from build123d import *

# Parameters (mm, degrees)
MODEL_R                 = 1.5
SALIENTE_EXTRUIR1_DEPTH = 3


with BuildPart() as part:
    # Model → Saliente-Extruir1 (new body)
    with BuildSketch(Plane.XY):
        with BuildLine():
            Line((256.429131311, 228.742243614), (355.429131311, 228.742243614))
            ThreePointArc((355.429131311, 228.742243614), (358.611111826, 227.424224129), (359.929131311, 224.242243614))
            Line((359.929131311, 224.242243614), (359.929131311, 215.242243614))
            ThreePointArc((359.929131311, 215.242243614), (358.611111826, 212.060263099), (355.429131311, 210.742243614))
            Line((355.429131311, 210.742243614), (256.429131311, 210.742243614))
            ThreePointArc((256.429131311, 210.742243614), (253.247150795, 212.060263099), (251.929131311, 215.242243614))
            Line((251.929131311, 215.242243614), (251.929131311, 224.242243614))
            ThreePointArc((251.929131311, 224.242243614), (253.247150795, 227.424224129), (256.429131311, 228.742243614))
        make_face()
        with Locations((337.429131311, 215.242243614)):
            Circle(MODEL_R, mode=Mode.SUBTRACT)
        with Locations((319.429131311, 215.242243614)):
            Circle(MODEL_R, mode=Mode.SUBTRACT)
        with Locations((328.429131311, 215.242243614)):
            Circle(MODEL_R, mode=Mode.SUBTRACT)
        with Locations((310.429131311, 215.242243614)):
            Circle(MODEL_R, mode=Mode.SUBTRACT)
        with Locations((292.429131311, 215.242243614)):
            Circle(MODEL_R, mode=Mode.SUBTRACT)
        with Locations((301.429131311, 215.242243614)):
            Circle(MODEL_R, mode=Mode.SUBTRACT)
        with Locations((274.429131311, 215.242243614)):
            Circle(MODEL_R, mode=Mode.SUBTRACT)
        with Locations((283.429131311, 215.242243614)):
            Circle(MODEL_R, mode=Mode.SUBTRACT)
        with Locations((265.429131311, 215.242243614)):
            Circle(MODEL_R, mode=Mode.SUBTRACT)
        with Locations((256.429131311, 215.242243614)):
            Circle(MODEL_R, mode=Mode.SUBTRACT)
        with Locations((346.429131311, 215.242243614)):
            Circle(MODEL_R, mode=Mode.SUBTRACT)
        with Locations((355.429131311, 215.242243614)):
            Circle(MODEL_R, mode=Mode.SUBTRACT)
        with BuildLine():
            Line((267.929131311, 222.617243614), (262.929131311, 222.617243614))
            ThreePointArc((262.929131311, 222.617243614), (262.398801225, 222.836913528), (262.179131311, 223.367243614))
            Line((262.179131311, 223.367243614), (262.179131311, 225.117243614))
            ThreePointArc((262.179131311, 225.117243614), (262.398801225, 225.6475737), (262.929131311, 225.867243614))
            Line((262.929131311, 225.867243614), (267.929131311, 225.867243614))
            ThreePointArc((267.929131311, 225.867243614), (268.459461397, 225.6475737), (268.679131311, 225.117243614))
            Line((268.679131311, 225.117243614), (268.679131311, 223.367243614))
            ThreePointArc((268.679131311, 223.367243614), (268.459461397, 222.836913528), (267.929131311, 222.617243614))
        make_face(mode=Mode.SUBTRACT)
        with BuildLine():
            Line((285.929131311, 222.617243614), (280.929131311, 222.617243614))
            ThreePointArc((280.929131311, 222.617243614), (280.398801225, 222.836913528), (280.179131311, 223.367243614))
            Line((280.179131311, 223.367243614), (280.179131311, 225.117243614))
            ThreePointArc((280.179131311, 225.117243614), (280.398801225, 225.6475737), (280.929131311, 225.867243614))
            Line((280.929131311, 225.867243614), (285.929131311, 225.867243614))
            ThreePointArc((285.929131311, 225.867243614), (286.459461397, 225.6475737), (286.679131311, 225.117243614))
            Line((286.679131311, 225.117243614), (286.679131311, 223.367243614))
            ThreePointArc((286.679131311, 223.367243614), (286.459461397, 222.836913528), (285.929131311, 222.617243614))
        make_face(mode=Mode.SUBTRACT)
        with BuildLine():
            Line((258.929131311, 222.617243614), (253.929131311, 222.617243614))
            ThreePointArc((253.929131311, 222.617243614), (253.398801225, 222.836913528), (253.179131311, 223.367243614))
            Line((253.179131311, 223.367243614), (253.179131311, 225.117243614))
            ThreePointArc((253.179131311, 225.117243614), (253.398801225, 225.6475737), (253.929131311, 225.867243614))
            Line((253.929131311, 225.867243614), (258.929131311, 225.867243614))
            ThreePointArc((258.929131311, 225.867243614), (259.459461397, 225.6475737), (259.679131311, 225.117243614))
            Line((259.679131311, 225.117243614), (259.679131311, 223.367243614))
            ThreePointArc((259.679131311, 223.367243614), (259.459461397, 222.836913528), (258.929131311, 222.617243614))
        make_face(mode=Mode.SUBTRACT)
        with BuildLine():
            Line((276.929131311, 222.617243614), (271.929131311, 222.617243614))
            ThreePointArc((271.929131311, 222.617243614), (271.398801225, 222.836913528), (271.179131311, 223.367243614))
            Line((271.179131311, 223.367243614), (271.179131311, 225.117243614))
            ThreePointArc((271.179131311, 225.117243614), (271.398801225, 225.6475737), (271.929131311, 225.867243614))
            Line((271.929131311, 225.867243614), (276.929131311, 225.867243614))
            ThreePointArc((276.929131311, 225.867243614), (277.459461397, 225.6475737), (277.679131311, 225.117243614))
            Line((277.679131311, 225.117243614), (277.679131311, 223.367243614))
            ThreePointArc((277.679131311, 223.367243614), (277.459461397, 222.836913528), (276.929131311, 222.617243614))
        make_face(mode=Mode.SUBTRACT)
        with BuildLine():
            Line((294.929131311, 222.617243614), (289.929131311, 222.617243614))
            ThreePointArc((289.929131311, 222.617243614), (289.398801225, 222.836913528), (289.179131311, 223.367243614))
            Line((289.179131311, 223.367243614), (289.179131311, 225.117243614))
            ThreePointArc((289.179131311, 225.117243614), (289.398801225, 225.6475737), (289.929131311, 225.867243614))
            Line((289.929131311, 225.867243614), (294.929131311, 225.867243614))
            ThreePointArc((294.929131311, 225.867243614), (295.459461397, 225.6475737), (295.679131311, 225.117243614))
            Line((295.679131311, 225.117243614), (295.679131311, 223.367243614))
            ThreePointArc((295.679131311, 223.367243614), (295.459461397, 222.836913528), (294.929131311, 222.617243614))
        make_face(mode=Mode.SUBTRACT)
        with BuildLine():
            Line((303.929131311, 222.617243614), (298.929131311, 222.617243614))
            ThreePointArc((298.929131311, 222.617243614), (298.398801225, 222.836913528), (298.179131311, 223.367243614))
            Line((298.179131311, 223.367243614), (298.179131311, 225.117243614))
            ThreePointArc((298.179131311, 225.117243614), (298.398801225, 225.6475737), (298.929131311, 225.867243614))
            Line((298.929131311, 225.867243614), (303.929131311, 225.867243614))
            ThreePointArc((303.929131311, 225.867243614), (304.459461397, 225.6475737), (304.679131311, 225.117243614))
            Line((304.679131311, 225.117243614), (304.679131311, 223.367243614))
            ThreePointArc((304.679131311, 223.367243614), (304.459461397, 222.836913528), (303.929131311, 222.617243614))
        make_face(mode=Mode.SUBTRACT)
        with BuildLine():
            Line((321.929131311, 222.617243614), (316.929131311, 222.617243614))
            ThreePointArc((316.929131311, 222.617243614), (316.398801225, 222.836913528), (316.179131311, 223.367243614))
            Line((316.179131311, 223.367243614), (316.179131311, 225.117243614))
            ThreePointArc((316.179131311, 225.117243614), (316.398801225, 225.6475737), (316.929131311, 225.867243614))
            Line((316.929131311, 225.867243614), (321.929131311, 225.867243614))
            ThreePointArc((321.929131311, 225.867243614), (322.459461397, 225.6475737), (322.679131311, 225.117243614))
            Line((322.679131311, 225.117243614), (322.679131311, 223.367243614))
            ThreePointArc((322.679131311, 223.367243614), (322.459461397, 222.836913528), (321.929131311, 222.617243614))
        make_face(mode=Mode.SUBTRACT)
        with BuildLine():
            Line((312.929131311, 222.617243614), (307.929131311, 222.617243614))
            ThreePointArc((307.929131311, 222.617243614), (307.398801225, 222.836913528), (307.179131311, 223.367243614))
            Line((307.179131311, 223.367243614), (307.179131311, 225.117243614))
            ThreePointArc((307.179131311, 225.117243614), (307.398801225, 225.6475737), (307.929131311, 225.867243614))
            Line((307.929131311, 225.867243614), (312.929131311, 225.867243614))
            ThreePointArc((312.929131311, 225.867243614), (313.459461397, 225.6475737), (313.679131311, 225.117243614))
            Line((313.679131311, 225.117243614), (313.679131311, 223.367243614))
            ThreePointArc((313.679131311, 223.367243614), (313.459461397, 222.836913528), (312.929131311, 222.617243614))
        make_face(mode=Mode.SUBTRACT)
        with BuildLine():
            Line((357.929131311, 222.617243614), (352.929131311, 222.617243614))
            ThreePointArc((352.929131311, 222.617243614), (352.398801225, 222.836913528), (352.179131311, 223.367243614))
            Line((352.179131311, 223.367243614), (352.179131311, 225.117243614))
            ThreePointArc((352.179131311, 225.117243614), (352.398801225, 225.6475737), (352.929131311, 225.867243614))
            Line((352.929131311, 225.867243614), (357.929131311, 225.867243614))
            ThreePointArc((357.929131311, 225.867243614), (358.459461397, 225.6475737), (358.679131311, 225.117243614))
            Line((358.679131311, 225.117243614), (358.679131311, 223.367243614))
            ThreePointArc((358.679131311, 223.367243614), (358.459461397, 222.836913528), (357.929131311, 222.617243614))
        make_face(mode=Mode.SUBTRACT)
        with BuildLine():
            Line((348.929131311, 222.617243614), (343.929131311, 222.617243614))
            ThreePointArc((343.929131311, 222.617243614), (343.398801225, 222.836913528), (343.179131311, 223.367243614))
            Line((343.179131311, 223.367243614), (343.179131311, 225.117243614))
            ThreePointArc((343.179131311, 225.117243614), (343.398801225, 225.6475737), (343.929131311, 225.867243614))
            Line((343.929131311, 225.867243614), (348.929131311, 225.867243614))
            ThreePointArc((348.929131311, 225.867243614), (349.459461397, 225.6475737), (349.679131311, 225.117243614))
            Line((349.679131311, 225.117243614), (349.679131311, 223.367243614))
            ThreePointArc((349.679131311, 223.367243614), (349.459461397, 222.836913528), (348.929131311, 222.617243614))
        make_face(mode=Mode.SUBTRACT)
        with BuildLine():
            Line((339.929131311, 222.617243614), (334.929131311, 222.617243614))
            ThreePointArc((334.929131311, 222.617243614), (334.398801225, 222.836913528), (334.179131311, 223.367243614))
            Line((334.179131311, 223.367243614), (334.179131311, 225.117243614))
            ThreePointArc((334.179131311, 225.117243614), (334.398801225, 225.6475737), (334.929131311, 225.867243614))
            Line((334.929131311, 225.867243614), (339.929131311, 225.867243614))
            ThreePointArc((339.929131311, 225.867243614), (340.459461397, 225.6475737), (340.679131311, 225.117243614))
            Line((340.679131311, 225.117243614), (340.679131311, 223.367243614))
            ThreePointArc((340.679131311, 223.367243614), (340.459461397, 222.836913528), (339.929131311, 222.617243614))
        make_face(mode=Mode.SUBTRACT)
        with BuildLine():
            Line((330.929131311, 222.617243614), (325.929131311, 222.617243614))
            ThreePointArc((325.929131311, 222.617243614), (325.398801225, 222.836913528), (325.179131311, 223.367243614))
            Line((325.179131311, 223.367243614), (325.179131311, 225.117243614))
            ThreePointArc((325.179131311, 225.117243614), (325.398801225, 225.6475737), (325.929131311, 225.867243614))
            Line((325.929131311, 225.867243614), (330.929131311, 225.867243614))
            ThreePointArc((330.929131311, 225.867243614), (331.459461397, 225.6475737), (331.679131311, 225.117243614))
            Line((331.679131311, 225.117243614), (331.679131311, 223.367243614))
            ThreePointArc((331.679131311, 223.367243614), (331.459461397, 222.836913528), (330.929131311, 222.617243614))
        make_face(mode=Mode.SUBTRACT)
    extrude(amount=SALIENTE_EXTRUIR1_DEPTH)


solid = part.part
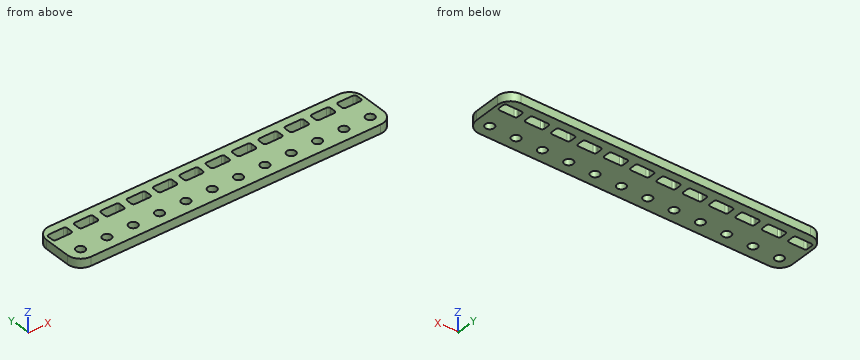
Source: CAD feature listing. Evaluate the final solid. Frame: model axes, mm. Give positions to 0.01 mm unless a question says otherwise; leave off trailing zeros. Write each loop counter-clockwise with the first axis right and the second up, starting at its lowest first coordinate (ties: lowest second). Pieces come first, ordered by that corner, then holes. Notation, with made-up numbers: M 12.5,6.25 L 21.5,6.25 A29 cw 21.5,28.25 Z; hole C 62.25,45 d11. An arc over 180 degrees is marked long. Return JSON: item names as keys, results as strings. Group by question number.
1) Cut plane B-B, the plane y = 227.25. Output: boundary loops of the cut face in (x, z).
2) Cut plane A-A, the plane z = 2.15. Give the number of separate pieces and of enclosed holes in the cut face, then the cut area to 3 significant figures.
3) Ray query, L1, parallel to Y at x = 328.5, z = 2.25; L2, parallel to Y at x = 335.5, z = 2.9; L3, parallel to Y at x = 302, z = 2.75. Return the intervals inside material, ascending.
Data:
{
 "1": {"outline": "M 253.08,0 L 358.78,0 L 358.78,3 L 253.08,3 Z"},
 "2": {"separate pieces": "1", "enclosed holes": "24", "area": "1,590 mm²"},
 "3": {"L1": "y = 210.74 to 213.74, 216.74 to 222.62, 225.87 to 228.74", "L2": "y = 210.74 to 222.62, 225.87 to 228.74", "L3": "y = 210.74 to 213.86, 216.63 to 222.62, 225.87 to 228.74"}
}
